Source: CAD feature listing. Evaluate the final solid. Frame: model axes, mm. A direction names the side the tool comes from. Give positions to 0.01 mm unless a question says otherwise; leave off trailing zeros. Order: outer loops, then holes, each group sorted by start corner. A loop starts at its lowest first (then second) coordinate and runs counter-clockwise, first axis right, second up.
from build123d import *

# Parameters (mm, degrees)
F1_DEPTH = 50
F2_R     = 7.5
F3_DEPTH = 50.001
F5_W     = 80
F5_H     = 15
F6_DEPTH = 15


with BuildPart() as f1:
    # F0 (on Front) → F1 (new body)
    with BuildSketch(Plane.XZ):
        Polygon((0, 45), (0, 0), (80, 0), (80, 25), (30, 45), align=None)
    extrude(amount=F1_DEPTH)

    # F2 (on face) → F3 (cut, through all)
    with BuildSketch(Plane.XZ.offset(50)):
        with Locations((20, 20)):
            Circle(F2_R)
    extrude(amount=-F3_DEPTH, mode=Mode.SUBTRACT)

    # F5 (on face) → F6 (cut, through all)
    with BuildSketch(Plane.XY.offset(45)):
        with Locations((40, -32.5)):
            Rectangle(F5_W, F5_H)
    extrude(amount=-F6_DEPTH, mode=Mode.SUBTRACT)


solid = f1.part
(1) Section A-A, the plane z = 20. Return loops of the section in (x, y).
(2) Section B-B, the plane x = 44.5. Return loops of the section in (y, z).
(3) Section D-D, the plane y = -4.5. Return loops of the section in (x, z), plus the area to 3 significant figures.
(4) Access query for faces 1 (the cylindrical face through (14.5, -25.4, 25.1)), 2 (the flat face through (26, -25, 36)). Directions: +Z, -Z, +X, -X, +Y, -Y. A direction counts if a zero-diameter tool reaches every point of the face in a straight line with its end or side. Return the directions, or none.
(5) Line query: line 1 along Y through (x, z) = (10, 37.5); line 2 along Z through (x, y) = (20, -22); line 3 along Z through (x, y) = (20, -30). Output: solid intervals per line, ascending.
(6) Draft query along Y for faces 3 (the flat face through (39, 0, 18)), 4 (the flat face through (39, -50, 18)), 5 (the flat face through (26, -40, 36)), 6 (the flat face through (80, -25, 12)). Return one class per face: +Y half, -Y half, draft (parallel to the pull), parting line (faces both ways), or undercut.
(7) Section C-C, the plane x = 20. Return loops of the section in (y, z).
(8) Pin query (flat end, axial travel): pin 1 Ø12 at (x, z) = (20, 20) entering from +Y; pin 2 Ø12 at (x, y) = (52, -43) entering from +Z; pin 3 Ø12 at (x, y) = (18, -31.5) entering from +Z. Return the tip coordinate at first contact, or that it passes through.
Checks:
1. outline: (0, -50) - (12.5, -50) - (12.5, 0) - (0, 0) - close; (27.5, -50) - (80, -50) - (80, 0) - (27.5, 0) - close
2. outline: (-50, 0) - (0, 0) - (0, 39.2) - (-25, 39.2) - (-25, 30) - (-40, 30) - (-40, 39.2) - (-50, 39.2) - close
3. outline: (0, 0) - (80, 0) - (80, 25) - (30, 45) - (0, 45) - close; hole circle Ø15 at (20, 20)
3. area: 2,920 mm2
4. face 1: +Y, -Y
4. face 2: +Z, +X, -X
5. line 1: y = -50 to -40, -25 to 0
5. line 2: z = 0 to 12.5, 27.5 to 45
5. line 3: z = 0 to 12.5, 27.5 to 30
6. face 3: +Y half
6. face 4: -Y half
6. face 5: undercut
6. face 6: draft
7. outline: (-50, 0) - (0, 0) - (0, 12.5) - (-50, 12.5) - close; (-50, 27.5) - (0, 27.5) - (0, 45) - (-25, 45) - (-25, 30) - (-40, 30) - (-40, 45) - (-50, 45) - close
8. pin 1: passes through
8. pin 2: stops at z = 38.6
8. pin 3: stops at z = 30
